from build123d import *

# Parameters (mm, degrees)
STOCK_SPINE_MASTER_1_START                   = -34.2
STOCK_SPINE_MASTER_1_OUTLINE_R               = 2.25
STOCK_SPINE_MASTER_1_OUTLINE_R_2             = 5.5
STOCK_SPINE_MASTER_1_DEPTH                   = 3.2
FILLET1_R                                    = 5
CUT_EXTRUDE2_DEPTH                           = 44.022458369
FILLET2_R                                    = 2
CSK_FOR_M4_COUNTERSUNK_FLAT_HEAD_SCR_2_COUNT = 2
CSK_FOR_M4_COUNTERSUNK_FLAT_HEAD_SCR_2_PITCH = 16
CSK_FOR_M4_COUNTERSUNK_FLAT_HEAD_SCR_3_COUNT = 2
CSK_FOR_M4_COUNTERSUNK_FLAT_HEAD_SCR_3_PITCH = 22.627416998
CSK_FOR_M4_COUNTERSUNK_FLAT_HEAD_SCR_4_COUNT = 2
CSK_FOR_M4_COUNTERSUNK_FLAT_HEAD_SCR_4_PITCH = 16


# Read off the part's stored shape, not the designer's step: Stock-spine_master-1
with BuildPart() as part:
    # Stock-spine_master-1 outline → Stock-spine_master-1 (new body)
    with BuildSketch(Plane.XY.offset(STOCK_SPINE_MASTER_1_START)):
        with BuildLine():
            Line((19.5, -38.215728753), (19.5, 0))
            ThreePointArc((19.5, 0), (0, 19.5), (-19.5, 0))
            Line((-19.5, 0), (-19.5, -38.215728753))
            Line((-19.5, -38.215728753), (19.5, -38.215728753))
        make_face()
        with Locations((0, -33)):
            Circle(STOCK_SPINE_MASTER_1_OUTLINE_R, mode=Mode.SUBTRACT)
        with Locations((-8, -8)):
            Circle(STOCK_SPINE_MASTER_1_OUTLINE_R, mode=Mode.SUBTRACT)
        with Locations((-8, 8)):
            Circle(STOCK_SPINE_MASTER_1_OUTLINE_R, mode=Mode.SUBTRACT)
        with Locations((8, -8)):
            Circle(STOCK_SPINE_MASTER_1_OUTLINE_R, mode=Mode.SUBTRACT)
        Circle(STOCK_SPINE_MASTER_1_OUTLINE_R_2, mode=Mode.SUBTRACT)
        with Locations((8, 8)):
            Circle(STOCK_SPINE_MASTER_1_OUTLINE_R, mode=Mode.SUBTRACT)
    extrude(amount=STOCK_SPINE_MASTER_1_DEPTH)

    # Fillet1
    fillet1_edges = [part.edges().sort_by_distance(p)[0] for p in [
        (-19.5, -38.215728753, -32.6),
        (19.5, -38.215728753, -32.6),
    ]]
    fillet(fillet1_edges, radius=FILLET1_R)

    # Sketch1 → Cut-Extrude2 (cut, through all)
    with BuildSketch(Plane.XY.offset(-31)):
        with BuildLine():
            ThreePointArc((13.5, -14.071247279), (8.649489408, -17.476736909), (3, -19.267848868))
            Line((3, -19.267848868), (3, -27.51707195))
            ThreePointArc((3, -27.51707195), (5.165471514, -29.481420167), (6.200598246, -32.215728753))
            Line((6.200598246, -32.215728753), (6.25, -32.215728753))
            Line((6.25, -32.215728753), (13.5, -32.215728753))
            Line((13.5, -32.215728753), (13.5, -14.071247279))
        make_face()
        with BuildLine():
            Line((-3, -27.51707195), (-3, -19.267848868))
            ThreePointArc((-3, -19.267848868), (-8.649489408, -17.476736909), (-13.5, -14.071247279))
            Line((-13.5, -14.071247279), (-13.5, -32.215728753))
            Line((-13.5, -32.215728753), (-6.25, -32.215728753))
            Line((-6.25, -32.215728753), (-6.200598246, -32.215728753))
            ThreePointArc((-6.200598246, -32.215728753), (-5.165471514, -29.481420167), (-3, -27.51707195))
        make_face()
    extrude(amount=-CUT_EXTRUDE2_DEPTH, mode=Mode.SUBTRACT)

    # Fillet2
    fillet2_edges = [part.edges().sort_by_distance(p)[0] for p in [
        (3, -19.267848868, -32.6),
        (13.5, -14.071247279, -32.6),
        (13.5, -32.215728753, -32.6),
        (-13.5, -14.071247279, -32.6),
        (-3, -19.267848868, -32.6),
        (-13.5, -32.215728753, -32.6),
    ]]
    fillet(fillet2_edges, radius=FILLET2_R)

    # Sketch4 → CSK for M4 Countersunk Flat Head Screw1 (revolve, cut)
    with BuildSketch(Plane(origin=(-8, -8, -31), x_dir=(0, -1, 0), z_dir=(1, 0, 0))):
        Polygon((0, 0), (0, 3.2), (2.25, 3.2), (2.25, 2.45), (4.7, 0), align=None)
    csk_for_m4_countersunk_flat_head_screw1 = revolve(axis=Axis((-8, -8, -24.65), (0, 0, -1)), mode=Mode.SUBTRACT)

    # CSK for M4 Countersunk Flat Head Scr 2: CSK for M4 Countersunk Flat Head Screw1 ×2
    with Locations(*[(i * CSK_FOR_M4_COUNTERSUNK_FLAT_HEAD_SCR_2_PITCH, 0, 0) for i in range(1, CSK_FOR_M4_COUNTERSUNK_FLAT_HEAD_SCR_2_COUNT)]):
        add(csk_for_m4_countersunk_flat_head_screw1, mode=Mode.SUBTRACT)

    # CSK for M4 Countersunk Flat Head Scr 3: CSK for M4 Countersunk Flat Head Screw1 ×2
    with Locations(*[Vector(0.7071067811865426, 0.7071067811865526, 0) * (i * CSK_FOR_M4_COUNTERSUNK_FLAT_HEAD_SCR_3_PITCH) for i in range(1, CSK_FOR_M4_COUNTERSUNK_FLAT_HEAD_SCR_3_COUNT)]):
        add(csk_for_m4_countersunk_flat_head_screw1, mode=Mode.SUBTRACT)

    # CSK for M4 Countersunk Flat Head Scr 4: CSK for M4 Countersunk Flat Head Screw1 ×2
    with Locations(*[(0, i * CSK_FOR_M4_COUNTERSUNK_FLAT_HEAD_SCR_4_PITCH, 0) for i in range(1, CSK_FOR_M4_COUNTERSUNK_FLAT_HEAD_SCR_4_COUNT)]):
        add(csk_for_m4_countersunk_flat_head_screw1, mode=Mode.SUBTRACT)


solid = part.part
The listing builds one solid part. Answer for the finished solid, in the listing's coordinates (mm). A direction names the side the tool comes from. Round coordinates to 2 decimals unless told otherwise and drop trailing zeros. Write each loop counter-clockwise with the first axis right and the second up, starting at its lowest first coordinate (ties: lowest second). Pieces come first, ordered by that corner, then holes. Notation, with made-up numbers: M 60.5,88.25 L 103.5,88.25 A27 cw 103.5,119.25 Z; hole C 9.25,65 d3. An arc over 180 degrees is marked long. Write each question's results on one line, items separated by ' | '. Start each with the question number.
Item 1: The mould has two halves that part along Y. Classify faces 3 (the cylindrical face through (0.429, 19.495, -32.622)), 4 (the cylindrical face through (-12.93, -31.614, -32.622)), 5 (the flat face through (0, -9, -31)), 6 (the cylindrical face through (18.074, -36.712, -32.578)): +Y half, -Y half, draft (parallel to the pull), parting line (faces both ways), or undercut.
Item 2: Which of the six approach directions +Z, -Z, +X, -X, +Y, -Y give full straight-line access (tool end or side, diameter ignored) to faces 1 (the flat face through (13.5, -24, -33)), 2 (the flat face through (19.5, -17, -33))?
Item 3: Straight lines are drawn through the part: probe 1 along X at (y, z) = (-8, -33.7); probe 2 along X at (y, z) = (-5, -32.1); probe 3 along X at (y, z) = (6, -33.7). For each, find the intervals that lie inside material, in ascending order.
Item 4: Find section D-D on y = -8. Write down the section's boundary in (x, z).
Item 5: Find section C-C on x = 0. Write down the section's boundary in (y, z), and give its area (3 significant figures).
Item 6: Given pin 1 Ø1 at (x, z) = (-10, -33) entering from +Y; pin 2 Ø1.6 at (x, z) = (9, -33.5) entering from +Y, each flat-ended and moving along its own axis, determine where each tip first touches the part or whether it passes through.
Item 7: Find section A-A on y = -23.5. Write down the section's boundary in (x, z), and give its area (3 significant figures).
Item 8: Find section B-B on z = -31.5. Give the number of separate pieces and of enclosed holes in the cut face, and give its area (3 significant figures).
Answer block:
1) face 3: +Y half | face 4: undercut | face 5: draft | face 6: -Y half
2) face 1: +Z, -Z | face 2: +Z, -Z, +X, +Y, -Y
3) probe 1: x = -19.5 to -10.25, -5.75 to 5.75, 10.25 to 19.5 | probe 2: x = -19.5 to -9.99, -6.01 to -2.29, 2.29 to 6.01, 9.99 to 19.5 | probe 3: x = -18.55 to -9.03, -6.97 to 6.97, 9.03 to 18.55
4) outline: M -19.5,-34.2 L -10.25,-34.2 L -10.25,-33.45 L -12.7,-31 L -19.5,-31 Z; M -5.75,-34.2 L 5.75,-34.2 L 5.75,-33.45 L 3.3,-31 L -3.3,-31 L -5.75,-33.45 Z; M 10.25,-34.2 L 19.5,-34.2 L 19.5,-31 L 12.7,-31 L 10.25,-33.45 Z
5) outline: M -38.22,-34.2 L -35.25,-34.2 L -35.25,-31 L -38.22,-31 Z; M -30.75,-34.2 L -5.5,-34.2 L -5.5,-31 L -30.75,-31 Z; M 5.5,-34.2 L 19.5,-34.2 L 19.5,-31 L 5.5,-31 Z | area: 135 mm²
6) pin 1: stops at y = 17.03 | pin 2: stops at y = 17.69
7) outline: M -19.5,-34.2 L -13.5,-34.2 L -13.5,-31 L -19.5,-31 Z; M -3,-34.2 L 3,-34.2 L 3,-31 L -3,-31 Z; M 13.5,-34.2 L 19.5,-34.2 L 19.5,-31 L 13.5,-31 Z | area: 57.6 mm²
8) separate pieces: 1 | enclosed holes: 8 | area: 1,460 mm²
